from build123d import *

# Parameters (mm, degrees)
F0_R     = 32.205
F1_DEPTH = 109.601
F2_R     = 9.525
F3_DEPTH = 3.9878
F4_R     = 3.9751
F5_DEPTH = 31.623
F7_DEPTH = 28.6004
F9_D     = 4.0386
F9_DEPTH = 12
F9_TIP   = 1.213317848


with BuildPart() as f1:
    # F0 (on Top) → F1 (new body)
    with BuildSketch(Plane.XY):
        Circle(F0_R)
    extrude(amount=F1_DEPTH)

    # F2 (on face) → F3 (join)
    with BuildSketch(Plane.XY.offset(109.601)):
        Circle(F2_R)
    extrude(amount=F3_DEPTH)

    # F4 (on face) → F5 (join)
    with BuildSketch(Plane.XY.offset(113.5888)):
        Circle(F4_R)
    extrude(amount=F5_DEPTH)

    # F6 (on face) → F7 (cut)
    with BuildSketch(Plane.XY.offset(145.2118)):
        with BuildLine():
            Line((0.9462931883, 2.5), (0.9462931883, 3.8608223492))
            ThreePointArc((0.9462931883, 3.8608223492), (-0.0554917727, 3.9747126529), (-1.0537068117, 3.8328999419))
            Line((-1.0537068117, 3.8328999419), (-1.0537068117, 2.5))
            Line((-1.0537068117, 2.5), (0.9462931883, 2.5))
        make_face()
    extrude(amount=-F7_DEPTH, mode=Mode.SUBTRACT)

    # F9
    with Locations(Plane.XY.offset(109.601)):
        with Locations((0.0541911848, 25.3999421912), (25.4, 0), (-25.4, 0), (0, -25.4)):
            Hole(F9_D / 2, depth=F9_DEPTH)
            with Locations((0, 0, -(F9_DEPTH + F9_TIP / 2))):  # 118° drill point
                Cone(0, F9_D / 2, F9_TIP, mode=Mode.SUBTRACT)


solid = f1.part
Work out the finished part from the listing and answer in its coordinate system (mm). A direction names the side the tool comes from. Give positions to 0.01 mm unless a question says otherwise; leave off trailing zeros. Write each loop counter-clockwise with the first axis right and the second up, starting at its lowest first coordinate (ties: lowest second). Pieces come first, ordered by that corner, then holes. Notation, with made-up numbers: (85.25, 70.25) - (124.25, 70.25) arc R30 ccw to (124.25, 103.25) - close; hole circle Ø11 at (72.25, 84.25). An arc over 180 degrees is marked (long way). One line per item, written item: value. Start each with the question number.
1. Consider probe 1 along Y at (x, z) = (0, 105.75) (3 decimals); probe 2 along Z at (x, y) = (12.5, -1); probe 3 along Z at (x, y) = (-5.5, 7). Determine where each line is inside the solid, lowest interval first.
2. For faces 1 (the cylindrical face through (-27.326, 0.607, 103.517)), 2 (the cylindrical face through (-6.98, -31.44, 54.03)), determine the directions among +Z, -Z, +X, -X, +Y, -Y from which every point of the face is accessible in a straight line to the end or side of a thin tool.
3. Find section D-D (z = 60). Write down the section's boundary in (x, y) (3 decimals), then the cut area to 3 significant figures.
4. For a pull along X with two mould halves and no side action, classify faces 3 (the conical face through (-0.076, -25.742, 96.598)), 4 (the flat face through (0, 0, 0)), 5 (the conical face through (-0.022, 25.058, 96.598)), 6 (the cylindrical face through (-7.559, -5.796, 111.567)) as +X half, -X half, draft (parallel to the pull), parting line (faces both ways), or undercut.
5. Find section C-C (x = -8). Write down the section's boundary in (y, z).
6. Find section B-B (y = 6). Write down the section's boundary in (x, z).
7. Find section A-A (z = 133.5). Write down the section's boundary in (x, y).
8. Given pin 1 (5 mm diameter, centred on y = 8, z = 22.5, fed in from +X); pin 2 (1 mm diameter, centred on x = 9, y = 15, fed in from +Z); pin 3 (3 mm diameter, centred on x = 19.5, z = 73, fed in from -Y); pin 4 (1.6 mm diameter, centred on x = 0, y = 3, fed in from +Z), each flat-ended and moving along its own axis, determine where each tip first touches the part or whether it passes through.
Geometry results:
1. probe 1: -32.205 to -27.419, -23.381 to 23.381, 27.419 to 32.205
1. probe 2: 0 to 109.6
1. probe 3: 0 to 113.59
2. face 1: +Z
2. face 2: +Z, -Z
3. outline: circle Ø64.41 at (0, 0)
3. area: 3,260 mm2
4. face 3: undercut
4. face 4: draft
4. face 5: undercut
4. face 6: parting line
5. outline: (-31.2, 0) - (31.2, 0) - (31.2, 109.6) - (5.17, 109.6) - (5.17, 113.59) - (-5.17, 113.59) - (-5.17, 109.6) - (-31.2, 109.6) - close
6. outline: (-31.64, 0) - (31.64, 0) - (31.64, 109.6) - (7.4, 109.6) - (7.4, 113.59) - (-7.4, 113.59) - (-7.4, 109.6) - (-31.64, 109.6) - close
7. outline: (-1.05, 2.5) - (-1.05, 3.83) arc R3.98 ccw (long way) to (0.95, 3.86) - (0.95, 2.5) - close
8. pin 1: x = 31.73
8. pin 2: z = 109.6
8. pin 3: y = -26.71
8. pin 4: z = 145.21
